Source: CAD feature listing. Evaluate the final solid. Frame: model axes, mm. A direction names the side the tool comes from. Give positions to 0.01 mm unless a question says otherwise; leave off trailing zeros. Order: outer loops, then holes, each group sorted by start corner. A loop starts at its lowest first (then second) coordinate and runs counter-clockwise, first axis right, second up. Notation, with made-up numbers: M -3,-2.5 L 33,-2.5 A35 cw 33,36.5 Z; hole C 69.25,-37.5 d2. An arc over 180 degrees is marked long. Return JSON: item names as keys, results as strings.
from build123d import *

# Parameters (mm, degrees)
SKETCH2_W           = 64.37
SKETCH2_H           = 29.59
BOSS_EXTRUDE1_DEPTH = 8
SKETCH3_W           = 3.485
SKETCH3_H           = 29.59
BOSS_EXTRUDE2_DEPTH = 50
FILLET2_R           = 3
SKETCH4_R           = 1.25
CUT_EXTRUDE8_DEPTH  = 70
SKETCH27_W          = 40.2
SKETCH27_H          = 3
CUT_EXTRUDE14_DEPTH = 12.295
SKETCH30_W          = 40.2
SKETCH30_H          = 3
CUT_EXTRUDE15_DEPTH = 12.295
SKETCH12_W          = 4
SKETCH12_H          = 3
CUT_EXTRUDE16_DEPTH = 60


with BuildPart() as part:
    # Sketch2 → Boss-Extrude1 (new body)
    with BuildSketch(Plane(origin=(0, 0, 0), x_dir=(1, 0, 0), z_dir=(0, 1, 0))):
        with Locations((-20.263080223, 14.424105874)):
            Rectangle(SKETCH2_W, SKETCH2_H)
    extrude(amount=BOSS_EXTRUDE1_DEPTH)

    # Sketch3 → Boss-Extrude2 (add)
    with BuildSketch(Plane(origin=(0, 8, 0), x_dir=(1, 0, 0), z_dir=(0, 1, 0))):
        with Locations((-50.705580223, 14.424105874)):
            Rectangle(SKETCH3_W, SKETCH3_H)
        with Locations((10.179419777, 14.424105874)):
            Rectangle(SKETCH3_W, SKETCH3_H)
    extrude(amount=BOSS_EXTRUDE2_DEPTH)

    # Fillet2
    fillet2_edges = [part.edges().sort_by_distance(p)[0] for p in [
        (11.921919777, 0, -14.424105874),
        (-52.448080223, 0, -14.424105874),
    ]]
    fillet(fillet2_edges, radius=FILLET2_R)

    # Sketch4 → Cut-Extrude8 (cut)
    with BuildSketch(Plane.ZY.offset(52.448080223)):
        with BuildLine():
            Line((-29.219105874, 8), (-25.296901218, 39.40325627))
            ThreePointArc((-25.296901218, 39.40325627), (-14.233202156, 50.466955332), (-3.169503094, 39.40325627))
            Line((-3.169503094, 39.40325627), (0.370894126, 8))
            Line((0.370894126, 8), (0.370894126, 58))
            Line((0.370894126, 58), (-29.219105874, 58))
            Line((-29.219105874, 58), (-29.219105874, 8))
        make_face()
        with Locations((-21.733202156, 42.90325627)):
            Circle(SKETCH4_R)
        with Locations((-21.733202156, 39.40325627)):
            Circle(SKETCH4_R)
        with Locations((-21.733202156, 35.90325627)):
            Circle(SKETCH4_R)
        with Locations((-17.733202156, 31.90325627)):
            Circle(SKETCH4_R)
        with Locations((-10.733202156, 31.90325627)):
            Circle(SKETCH4_R)
        with Locations((-6.733202156, 35.90325627)):
            Circle(SKETCH4_R)
        with Locations((-6.733202156, 39.40325627)):
            Circle(SKETCH4_R)
        with Locations((-6.733202156, 42.90325627)):
            Circle(SKETCH4_R)
        with Locations((-10.733202156, 46.90325627)):
            Circle(SKETCH4_R)
        with Locations((-17.733202156, 46.90325627)):
            Circle(SKETCH4_R)
        with Locations((-14.233202156, 46.90325627)):
            Circle(SKETCH4_R)
        with Locations((-14.233202156, 31.90325627)):
            Circle(SKETCH4_R)
    extrude(amount=-CUT_EXTRUDE8_DEPTH, mode=Mode.SUBTRACT)

    # Sketch27 → Cut-Extrude14 (cut)
    with BuildSketch(Plane.XY.offset(0.370894126)):
        with Locations((-20.263080223, 4)):
            Rectangle(SKETCH27_W, SKETCH27_H)
    extrude(amount=-CUT_EXTRUDE14_DEPTH, mode=Mode.SUBTRACT)

    # Sketch30 → Cut-Extrude15 (cut)
    with BuildSketch(Plane(origin=(0, 0, -29.219105874), x_dir=(-1, 0, 0), z_dir=(0, 0, -1))):
        with Locations((20.263080223, 4)):
            Rectangle(SKETCH30_W, SKETCH30_H)
    extrude(amount=-CUT_EXTRUDE15_DEPTH, mode=Mode.SUBTRACT)

    # Sketch12 → Cut-Extrude16 (cut)
    with BuildSketch(Plane(origin=(11.921919777, 0, 0), x_dir=(0, 0, -1), z_dir=(1, 0, 0))):
        with Locations((12.424105874, 16.5)):
            Rectangle(SKETCH12_W, SKETCH12_H)
        with Locations((16.424105874, 16.5)):
            Rectangle(SKETCH12_W, SKETCH12_H)
    extrude(amount=-CUT_EXTRUDE16_DEPTH, mode=Mode.SUBTRACT)


solid = part.part
1. Section query B-B (z = -14). State how many separate pieces and enclosed holes the cut face has, then the cut area to 3 significant figures.
Evaluation:
{"separate pieces": "6", "enclosed holes": "0", "area": "762 mm^2"}
2. Set-up query: faces 5 (the face through (-0.163, 4, -23)), 6 (the face through (10, 15, -14)), 7 (the face through (-50.73, 38.183, -22.004)). Return all of +Z, -Z, +X, -X, +Y, -Y with unobstructed straight access to the full face (end or side cutting, diameter ignored); none if empty.
Evaluation:
{"face 5": "-Z", "face 6": "+X", "face 7": "+X, -X"}
3. Section query C-C (y = 17). Return loops of the section in (x, z).
Evaluation:
{"outline": "M -52.45,-28.1 L -48.96,-28.1 L -48.96,-0.64 L -52.45,-0.64 Z; M 8.44,-28.1 L 11.92,-28.1 L 11.92,-18.42 L 8.44,-18.42 Z; M 8.44,-10.42 L 11.92,-10.42 L 11.92,-0.64 L 8.44,-0.64 Z"}
4. Draft query along Y for faces 1 (the face through (10.16, 46.96, -18.98)), 2 (the face through (-50.73, 45.794, -10.156)), 3 (the face through (10.155, 23.482, -27.285)), 4 (the face through (-48.963, 24, -14)). Return one class per face: pulls with the +Y half, pulls with the -Y half, needs draft (parallel to the pull), parting line crosses it, or undercut.
Evaluation:
{"face 1": "undercut", "face 2": "undercut", "face 3": "pulls with the +Y half", "face 4": "needs draft"}
5. Section query D-D (y = 4). Return loops of the section in (x, z).
Evaluation:
{"outline": "M -52.45,-29.22 L -40.36,-29.22 L -40.36,-16.92 L -0.16,-16.92 L -0.16,-29.22 L 11.92,-29.22 L 11.92,0.37 L -0.16,0.37 L -0.16,-11.92 L -40.36,-11.92 L -40.36,0.37 L -52.45,0.37 Z"}
6. Section query A-A (x = -18.5). Return loops of the section in (y, z), then the cut area to 3 significant figures.
Evaluation:
{"outline": "M 0,-29.22 L 2.5,-29.22 L 2.5,-16.92 L 5.5,-16.92 L 5.5,-29.22 L 8,-29.22 L 8,0.37 L 5.5,0.37 L 5.5,-11.92 L 2.5,-11.92 L 2.5,0.37 L 0,0.37 Z", "area": "163 mm^2"}
7. Ray query, probe 1 along Y at (x, z) = (-30, -25); probe 2 along X at (y, z) = (44.5, -17.75); probe 3 along Y at (x, z) = (-41.5, -25.25). Return the intervals inside material, ascending.
Evaluation:
{"probe 1": "y = 0 to 2.5, 5.5 to 8", "probe 2": "x = -52.45 to -48.96, 8.44 to 11.92", "probe 3": "y = 0 to 8"}
8. First-contact query: pin 1 (3 mm diameter, centred on y = 46.9, z = -14.23, fed in from +X); pin 2 (1.5 mm diameter, centred on x = -16.5, y = 3.5, fed in from -Z); pin 3 (3.5 mm diameter, centred on x = 11, y = 16.5, fed in from -Z); pin 4 (1.7 mm diameter, centred on x = 10, z = -14, fed in from -Y). Flat tips, straight axial feed; report the tip coordinate or a pass-through.
Evaluation:
{"pin 1": "stops at x = 11.92", "pin 2": "stops at z = -16.92", "pin 3": "stops at z = -28.38", "pin 4": "stops at y = 0.01"}
